Read the model definition and answer for the solid it produces. Units are mm, in the model's axes. A direction names the side the tool comes from. Round coordinates to 2 decimals unless told otherwise and drop trailing zeros. Write each loop counter-clockwise with the first axis right and the second up, starting at its lowest first coordinate (ties: lowest second). Pieces come first, ordered by that corner, then holes. Notation, with made-up numbers: (-16, 11.25) -> (5, 11.25) arc R29 ccw to (5, 31.25) -> close; hole circle Ø11 at (89, 66). An arc over 180 degrees is marked (long way). Return JSON: item names as keys, results as strings. Group by question number.
(1) A cutting plane is placed at C-C on y = -6.25. Give the vertices of the cut face in (x, z) (3 decimals), then the cut area to 3 significant figures.
(2) For faces 4 (the flat face through (-1.024, -11.135, -1.79)), 5 (the flat face through (1, -12.7, -2)), determine the directions among +Z, -Z, +X, -X, +Y, -Y from which every point of the face is accessible in a straight line to the end or side of a thin tool.
(3) A cutting plane is placed at A-A on y = -11.5. Give the vertices of the cut face in (x, z) (3 decimals), then the cut area to 3 significant figures.
(4) A cutting plane is placed at B-B on x = -1.25. Give the vertices of the cut face in (y, z) (3 decimals).
(5) Given pin 1 (3 mm diameter, centred on y = -9, z = -2.5, fed in from +X), flat-ended and moving along its own axis, determine where the tip first touches the part or whether it passes through.
(6) Straight lines are drawn through the part: line 1 (Y direction, x = 2, z = 0.5) (3 decimals); line 2 (X direction, y = -11.5, z = -2); line 3 (X direction, y = -9, z = 0.75). For each, find the intervals that lie inside material, in ascending order.
(7) A cutting plane is placed at D-D on z = 0.25. Give the vertices of the cut face in (x, y) (3 decimals).
(8) The mould has two halves that part along Z. Classify faces 1 (the cylindrical face through (-0.69, -6.26, -3.1)), 2 (the flat face through (0, 0, 0)), 3 (the flat face through (1.024, -11.135, 1.79)): released by +Z, released by -Z, zero draft, split by the parting line, or undercut.
```python
from build123d import *

# Parameters (mm, degrees)
F0_R     = 3.175
F1_DEPTH = 12.7
F3_DEPTH = 3.175
F4_DEPTH = 2.38125


with BuildPart() as f1:
    # F0 (on Front) → F1 (new body)
    with BuildSketch(Plane.XZ):
        Circle(F0_R)
    extrude(amount=F1_DEPTH)

    # F2 (on face) → F3 (cut)
    with BuildSketch(Plane.XZ.offset(12.7)):
        Polygon((-0.028336, 2.381081), (-2.076245, 1.166001), (-2.047909, -1.215081), (0.028336, -2.381081), (2.076245, -1.166001), (2.047909, 1.215081), align=None)
    extrude(amount=-F3_DEPTH, mode=Mode.SUBTRACT)

    # F2 (on face) → F4 (cut)
    with BuildSketch(Plane.XZ.offset(12.7)):
        Polygon((-0.028336, 2.381081), (-2.076245, 1.166001), (-2.047909, -1.215081), (0.028336, -2.381081), (2.076245, -1.166001), (2.047909, 1.215081), align=None)
    extrude(amount=-F4_DEPTH, mode=Mode.SUBTRACT)


solid = f1.part
```
Checks:
{
 "1": {"outline": "circle Ø6.35 at (0, 0)", "area": "31.7 mm^2"},
 "2": {"face 4": "-Y", "face 5": "+Z, -Z, +X, -X, -Y"},
 "3": {"outline": "circle Ø6.35 at (0, 0); hole (-2.076, 1.166) -> (-2.048, -1.215) -> (0.028, -2.381) -> (2.076, -1.166) -> (2.048, 1.215) -> (-0.028, 2.381) -> close", "area": "16.9 mm^2"},
 "4": {"outline": "(-12.7, -2.919) -> (0, -2.919) -> (0, 2.919) -> (-12.7, 2.919) -> (-12.7, 1.656) -> (-9.525, 1.656) -> (-9.525, -1.663) -> (-12.7, -1.663) -> close"},
 "5": {"pin 1": "stops at x = 3.01"},
 "6": {"line 1": "y = -9.525 to 0", "line 2": "x = -2.47 to -0.65, 0.67 to 2.47", "line 3": "x = -3.09 to 3.09"},
 "7": {"outline": "(-3.165, -12.7) -> (-2.065, -12.7) -> (-2.065, -9.525) -> (2.059, -9.525) -> (2.059, -12.7) -> (3.165, -12.7) -> (3.165, 0) -> (-3.165, 0) -> close"},
 "8": {"face 1": "split by the parting line", "face 2": "zero draft", "face 3": "undercut"}
}
